The model under review builds one solid part; all positions refer to its coordinate system, in mm. Face numbers are marked on the shaded views. A direction names the side the tool comes from. Give positions to 0.01 mm unless a question says otherwise; leave off trailing zeros. Order: outer loops, then holes, each group sorted by start corner. A loop starts at its lowest first (then second) coordinate and runs counter-clockwise, first axis right, second up.
```python
from build123d import *
from build123d.topology import SkipClean

# Parameters (mm, degrees)
EXTRUDE_1_DEPTH          = 12
PATTERN_CIRCULAR_1_COUNT = 4
RIB_1_REACH              = 114.643
SKETCH_4_WALL_W          = 251.024101548
SKETCH_4_WALL_H          = 1
PATTERN_CIRCULAR_2_COUNT = 8
SKETCH_6_R               = 3.4
CUT_EXTRUDE_1_DEPTH      = 105.276075876
SKETCH_7_R               = 6.25
CUT_EXTRUDE_2_DEPTH      = 2
PATTERN_CIRCULAR_3_COUNT = 4
SKETCH_8_R               = 2
CUT_EXTRUDE_3_DEPTH      = 105.276075876
PATTERN_CIRCULAR_4_COUNT = 4
EXTRUDE_START            = 1
SKETCH_9_R               = 5.25
SKETCH_9_R_2             = 3.4
EXTRUDE_2_DEPTH          = 1
PATTERN_CIRCULAR_5_COUNT = 4


with BuildPart() as part:
    # 草图1 → 旋转1 (revolve)
    with BuildSketch(Plane(origin=(0, 0, 0), x_dir=(0, 0, -1), z_dir=(1, 0, 0)), mode=Mode.PRIVATE) as revolve_1_sk:
        Polygon((0, 10.5), (0, 15), (28, 15), (28, 24), (25, 24), (25, 26), (30, 26), (43, 37.5), (43, 42.5), (48, 42.5), (48, 63.5), (59, 63.5), (59, 61.5), (53, 61.5), (53, 40.5), (45, 40.5), (45, 37.5), (56, 37.5), (56, 35.5), (43.757661732, 35.5), (30, 23.329760776), (30, 12), (51, 12), (51, 8.5), (14, 8.5), (14, 10.5), align=None)
    revolve(revolve_1_sk.sketch.rotate(Axis((0, 0, 0), (0, 0, -1)), 90), axis=Axis((0, 0, 0), (0, 0, -1)))

    # 草图3 → 凸台-拉伸1 (add)
    with BuildSketch(Plane(origin=(0, 0, -56), x_dir=(-1, 0, 0), z_dir=(0, 0, -1))):
        with BuildLine():
            Line((0, -37.5), (0, -35.5))
            ThreePointArc((0, -35.5), (-2.506253606, -35.411420373), (-5, -35.146123542))
            Line((-5, -35.146123542), (-5, -37.165171868))
            ThreePointArc((-5, -37.165171868), (-2.505599224, -37.416199333), (0, -37.5))
        make_face()
        with BuildLine():
            ThreePointArc((5, -35.146123542), (2.506253606, -35.411420373), (0, -35.5))
            Line((0, -35.5), (0, -37.5))
            ThreePointArc((0, -37.5), (2.505599224, -37.416199333), (5, -37.165171868))
            Line((5, -37.165171868), (5, -35.146123542))
        make_face()
    extrude_1 = extrude(amount=EXTRUDE_1_DEPTH)

    # 阵列(圆周)1: 凸台-拉伸1 ×4 about axis
    with SkipClean():  # the faces are left unmerged after this step: merging them gives an invalid solid
        pattern_circular_1_axis = Axis((0, 0, 0), (0, 0, 1))
        for i in range(1, PATTERN_CIRCULAR_1_COUNT):
            add(extrude_1.rotate(pattern_circular_1_axis, i * 360 / PATTERN_CIRCULAR_1_COUNT))

    # 草图4 wall → 筋1 (add, up to next)
    with BuildSketch(Plane(origin=(-23.810679894, 0, -50), x_dir=(-1, 0, 0), z_dir=(0, 0, 1)), mode=Mode.PRIVATE) as rib_1_sk1:
        Rectangle(SKETCH_4_WALL_W, SKETCH_4_WALL_H)
    rib_1_tool1 = extrude(rib_1_sk1.sketch, amount=RIB_1_REACH, mode=Mode.PRIVATE) - part.part
    rib_1 = rib_1_tool1.solids().sort_by_distance((-23.810679894, 0, -50))[0]
    add(rib_1)

    # 阵列(圆周)2: 筋1 ×8 about axis
    with SkipClean():  # the faces are left unmerged after this step: merging them gives an invalid solid
        pattern_circular_2_axis = Axis((0, 0, 0), (0, 0, 1))
        for i in range(1, PATTERN_CIRCULAR_2_COUNT):
            add(rib_1.rotate(pattern_circular_2_axis, i * 360 / PATTERN_CIRCULAR_2_COUNT))

    # 草图6 → 切除-拉伸1 (cut, symmetric)
    with SkipClean():  # the faces are left unmerged after this step: merging them gives an invalid solid
        with BuildSketch(Plane(origin=(0, 0, -53), x_dir=(-1, 0, 0), z_dir=(0, 0, -1))):
            with Locations((0, 54)):
                Circle(SKETCH_6_R)
        cut_extrude_1 = extrude(amount=CUT_EXTRUDE_1_DEPTH, both=True, mode=Mode.SUBTRACT)

    # 草图7 → 切除-拉伸2 (cut)
    with SkipClean():  # the faces are left unmerged after this step: merging them gives an invalid solid
        with BuildSketch(Plane.XY.offset(-48)):
            with Locations((0, 54)):
                Circle(SKETCH_7_R)
        cut_extrude_2 = extrude(amount=-CUT_EXTRUDE_2_DEPTH, mode=Mode.SUBTRACT)

    # 阵列(圆周)3: 切除-拉伸1, 切除-拉伸2 ×4 about axis
    with SkipClean():  # the faces are left unmerged after this step: merging them gives an invalid solid
        pattern_circular_3_axis = Axis((0, 0, 0), (0, 0, 1))
        add([cut_extrude_1.rotate(pattern_circular_3_axis, i * 360 / PATTERN_CIRCULAR_3_COUNT) for i in range(1, PATTERN_CIRCULAR_3_COUNT)], mode=Mode.SUBTRACT)
        add([cut_extrude_2.rotate(pattern_circular_3_axis, i * 360 / PATTERN_CIRCULAR_3_COUNT) for i in range(1, PATTERN_CIRCULAR_3_COUNT)], mode=Mode.SUBTRACT)

    # 草图8 → 切除-拉伸3 (cut, through all)
    with SkipClean():  # the faces are left unmerged after this step: merging them gives an invalid solid
        with BuildSketch(Plane(origin=(0, 0, -53), x_dir=(-1, 0, 0), z_dir=(0, 0, -1))):
            with Locations((38.183766184, 38.183766184)):
                Circle(SKETCH_8_R)
        cut_extrude_3 = extrude(amount=-CUT_EXTRUDE_3_DEPTH, mode=Mode.SUBTRACT)

    # 阵列(圆周)4: 切除-拉伸3 ×4 about axis
    with SkipClean():  # the faces are left unmerged after this step: merging them gives an invalid solid
        pattern_circular_4_axis = Axis((0, 0, 0), (0, 0, 1))
        for i in range(1, PATTERN_CIRCULAR_4_COUNT):
            add(cut_extrude_3.rotate(pattern_circular_4_axis, i * 360 / PATTERN_CIRCULAR_4_COUNT), mode=Mode.SUBTRACT)

    # 草图9 → 凸台-拉伸2 (add)
    with SkipClean():  # the faces are left unmerged after this step: merging them gives an invalid solid
        with BuildSketch(Plane(origin=(0, 0, -53), x_dir=(-1, 0, 0), z_dir=(0, 0, -1)).offset(EXTRUDE_START)):
            with Locations(Location((0, 54, 0), (0, 0, 180))):
                Circle(SKETCH_9_R)
            with Locations((0, 54)):
                Circle(SKETCH_9_R_2, mode=Mode.SUBTRACT)
        extrude_2 = extrude(amount=-EXTRUDE_2_DEPTH)

    # 阵列(圆周)5: 凸台-拉伸2 ×4 about axis
    with SkipClean():  # the faces are left unmerged after this step: merging them gives an invalid solid
        pattern_circular_5_axis = Axis((0, 0, 0), (0, 0, 1))
        for i in range(1, PATTERN_CIRCULAR_5_COUNT):
            add(extrude_2.rotate(pattern_circular_5_axis, i * 360 / PATTERN_CIRCULAR_5_COUNT))


solid = part.part
```
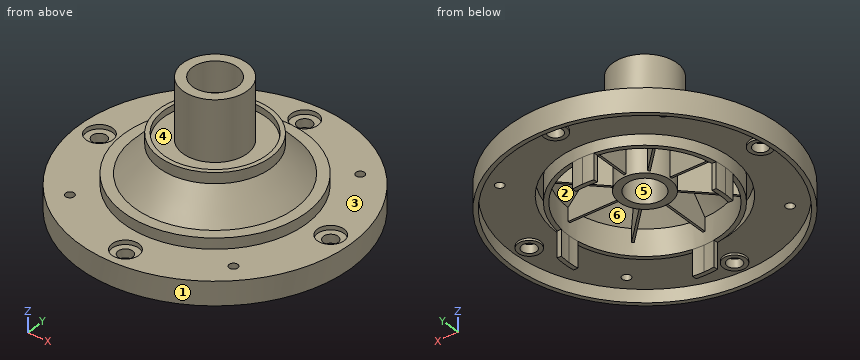
Item 1: For line 1 (Y direction, x = 0, z = -18); line 2 (Z direction, x = -17.5, y = 48.5); line 3 (Z direction, x = 41.5, y = 5), list the stretches that pass through material, from the lowest coordinate up.
Values found:
line 1: y = -15 to -8.5, 8.5 to 15
line 2: z = -53 to -48
line 3: z = -53 to -43
Item 2: Take a section at A-A (x = -54). Give the boundary of the cut face in (y, z), and give its area (3 significant figures).
Values found:
outline: (-33.41, -59) - (-29.43, -59) - (-29.43, -53) - (-5.25, -53) - (-5.25, -54) - (-3.4, -54) - (-3.4, -50) - (-6.25, -50) - (-6.25, -48) - (-33.41, -48) - close; (3.4, -54) - (5.25, -54) - (5.25, -53) - (29.43, -53) - (29.43, -59) - (33.41, -59) - (33.41, -48) - (6.25, -48) - (6.25, -50) - (3.4, -50) - close
area: 340 mm2
Item 3: Clearance check with flat-ended pins moving along their axes: pin 1 Ø5 at (x, y) = (-16, 16.5) entering from -Z; pin 2 Ø4.5 at (x, y) = (-8.5, -14) entering from -Z; pin 3 Ø10 at (x, y) = (45, -8) entering from +Z. State where each tip first meets the part, or that it passes through.
Values found:
pin 1: stops at z = -50
pin 2: stops at z = -30
pin 3: stops at z = -43
Item 4: Take a section at B-B (z = -35.5). Give the number of separate pieces and of enclosed holes in the cut face, and give its area (3 significant figures).
Values found:
separate pieces: 1
enclosed holes: 9
area: 850 mm2
Item 5: For the marked faces 4, 5 and 6, list the 3-axis set-ups (+Z, -Z, +X, -X, +Y, -Y) from which the entire face can be reached by the end or side of a thin tool; tool diameter is ignored.
Values found:
face 4: +Z
face 5: +Z, -Z
face 6: -Z
Item 6: Draft analysis for pull direction Y (two halves, no side actions). For the marked faces 1, 2 and 3, state which applies: released by +Y, released by -Y, zero draft, split by the parting line, or undercut.
Values found:
face 1: split by the parting line
face 2: undercut
face 3: zero draft
